Geometry: final body of the model. Coordinates: model frame, mm. Face numbers are marked on the shaded views. A direction names the side the tool comes from. Give positions to 0.01 mm unless a question says otherwise; leave off trailing zeros. Order: outer loops, then holes, each group sorted by start corner. A loop starts at its lowest first (then second) coordinate and runs counter-clockwise, first axis right, second up. Notation, with made-up numbers: (24.5, -25) - (63.5, -25) arc R27 ccw to (63.5, 10) - close; hole circle Ø5 at (50.5, 7). An arc over 180 degrees is marked (long way). Put each result on its own line as item: value. Start each with the question number.
1. Section C-C on y = -3.75. Return the cut outline in (x, z).
2. Set-up query: the marked faces 1 and 2. Return all of +Z, -Z, +X, -X, +Y, -Y with unobstructed straight access to the full face (end or side cutting, diameter ignored); none if empty.
3. First-contact query: P1, Ø1.5, axis at x = -2.5, y = -2, coming from the +Z side; P2, Ø3, axis at x = -2, y = -1, coming from the +Z side; P3, Ø2, axis at x = 2.5, z = -1.5, coming from the +Y side. Flat tips, straight axial feed; report the tip coordinate or a pass-through.
4. Section B-B on z = 0. Return the cut outline in (x, y), plus the area to 3 significant figures.
5. Section A-A on z = -5.5. Return the cut outline in (x, y), plus the area to 3 significant figures.
6. Ray query, line 1 along X through (y, z) = (-0.6, -2.25); line 2 along Y through (x, z) = (-2.75, 0). Return the intervals inside material, ascending. Write a range as from..to.
from build123d import *

# Parameters (mm, degrees)
F0_R      = 5.25
F1_DEPTH  = 4.6
F2_R      = 0.508
F4_DEPTH  = 0.2
F6_DEPTH  = 0.2
F7_W      = 0.2
F7_H      = 1
F8_DEPTH  = 1.7
F10_DEPTH = 0.2
F12_DEPTH = 0.2


with BuildPart() as f1:
    # F0 (on Front) → F1 (new body)
    with BuildSketch(Plane.XZ):
        Circle(F0_R)
    extrude(amount=F1_DEPTH)

    # F2
    f2_edges = [f1.edges().sort_by_distance(p)[0] for p in [
        (-5.25, -4.6, 0),
        (-5.25, 0, 0),
    ]]
    fillet(f2_edges, radius=F2_R)

    # F3 (on face) → F4 (join)
    with BuildSketch(Plane(origin=(0, 0, 0), x_dir=(-1, 0, 0), z_dir=(0, 1, 0))):
        with BuildLine():
            Line((0.8581771286, 0.338), (-0.8418228714, 0.338))
            Line((-0.8418228714, 0.338), (-0.8418228714, -4.6666795747))
            ThreePointArc((-0.8418228714, -4.6666795747), (-0.4225928635, -4.7231323581), (0, -4.742))
            ThreePointArc((0, -4.742), (0.430870892, -4.7223843844), (0.8581771286, -4.6636998205))
            Line((0.8581771286, -4.6636998205), (0.8581771286, 0.338))
        make_face()
        with BuildLine():
            ThreePointArc((0, -4.742), (-0.4225928635, -4.7231323581), (-0.8418228714, -4.6666795747))
            Line((-0.8418228714, -4.6666795747), (-0.8418228714, -4.742))
            Line((-0.8418228714, -4.742), (0, -4.742))
        make_face()
        with BuildLine():
            Line((0.8581771286, -4.742), (0.8581771286, -4.6636998205))
            ThreePointArc((0.8581771286, -4.6636998205), (0.430870892, -4.7223843844), (0, -4.742))
            Line((0, -4.742), (0.8581771286, -4.742))
        make_face()
    extrude(amount=F4_DEPTH)

    # F5 (on face) → F6 (join)
    with BuildSketch(Plane.XZ.offset(4.6)):
        with BuildLine():
            Line((-0.8581771286, -4.742), (0, -4.742))
            ThreePointArc((0, -4.742), (-0.430870892, -4.7223843844), (-0.8581771286, -4.6636998205))
            Line((-0.8581771286, -4.6636998205), (-0.8581771286, -4.742))
        make_face()
        with BuildLine():
            Line((0.8418228714, -4.6666795747), (0.8418228714, 0.338))
            Line((0.8418228714, 0.338), (-0.8581771286, 0.338))
            Line((-0.8581771286, 0.338), (-0.8581771286, -4.6636998205))
            ThreePointArc((-0.8581771286, -4.6636998205), (-0.430870892, -4.7223843844), (0, -4.742))
            ThreePointArc((0, -4.742), (0.4225928635, -4.7231323581), (0.8418228714, -4.6666795747))
        make_face()
        with BuildLine():
            Line((0.8418228714, -4.742), (0.8418228714, -4.6666795747))
            ThreePointArc((0.8418228714, -4.6666795747), (0.4225928635, -4.7231323581), (0, -4.742))
            Line((0, -4.742), (0.8418228714, -4.742))
        make_face()
    extrude(amount=F6_DEPTH)

    # F7 (on face) → F8 (join, through all)
    with BuildSketch(Plane.YZ.offset(0.8418228714)):
        with Locations((-4.8, -5.75)):
            Rectangle(F7_W, F7_H)
        with BuildLine():
            add(Edge.make_bspline(
                [(-4.8, -4.742), (-4.8333333333, -4.9113333333), (-4.901335109, -4.936598707), (-4.9, -5.25)],
                knots=[0, 0, 0, 0, 0.5177489739, 0.5177489739, 0.5177489739, 0.5177489739], degree=3))
            Line((-4.9, -5.25), (-4.7, -5.25))
            add(Edge.make_bspline(
                [(-4.6, -4.742), (-4.6333333333, -4.9113333333), (-4.7159921378, -4.9838428386), (-4.7, -5.25)],
                knots=[0, 0, 0, 0, 0.5177489739, 0.5177489739, 0.5177489739, 0.5177489739], degree=3))
            Line((-4.6, -4.742), (-4.8, -4.742))
        make_face()
        with Locations((0.2, -5.75)):
            Rectangle(F7_W, F7_H)
        with BuildLine():
            add(Edge.make_bspline(
                [(0, -4.742), (0.0333333333, -4.9113333333), (0.1159921378, -4.9838428386), (0.1, -5.25)],
                knots=[0, 0, 0, 0, 0.5177489739, 0.5177489739, 0.5177489739, 0.5177489739], degree=3))
            Line((0.1, -5.25), (0.3, -5.25))
            add(Edge.make_bspline(
                [(0.2, -4.742), (0.2333333333, -4.9113333333), (0.301335109, -4.936598707), (0.3, -5.25)],
                knots=[0, 0, 0, 0, 0.5177489739, 0.5177489739, 0.5177489739, 0.5177489739], degree=3))
            Line((0.2, -4.742), (0, -4.742))
        make_face()
    extrude(amount=-F8_DEPTH)

    # F9 (on face) → F10 (join, through all)
    with BuildSketch(Plane(origin=(0, 0.3, 0), x_dir=(-1, 0, 0), z_dir=(0, 1, 0))):
        with BuildLine():
            Line((0.4, -6.25), (-0.4, -6.25))
            Line((-0.4, -6.25), (-0.8418228714, -6.25))
            Line((-0.8418228714, -6.25), (-0.4735729361, -6.4726176162))
            ThreePointArc((-0.4735729361, -6.4726176162), (-0.4196612114, -6.5281834474), (-0.4, -6.6030665057))
            Line((-0.4, -6.6030665057), (-0.4, -9.0975669799))
            ThreePointArc((-0.4, -9.0975669799), (-0.3553534021, -9.2053534021), (-0.2475669799, -9.25))
            Line((-0.2475669799, -9.25), (0.2475669799, -9.25))
            ThreePointArc((0.2475669799, -9.25), (0.3553534021, -9.2053534021), (0.4, -9.0975669799))
            Line((0.4, -9.0975669799), (0.4, -6.6030665057))
            ThreePointArc((0.4, -6.6030665057), (0.4196612114, -6.5281834474), (0.4735729361, -6.4726176162))
            Line((0.4735729361, -6.4726176162), (0.8418228714, -6.25))
            Line((0.8418228714, -6.25), (0.4, -6.25))
        make_face()
    extrude(amount=-F10_DEPTH)

    # F11 (on face) → F12 (join, through all)
    with BuildSketch(Plane.XZ.offset(4.9)):
        with BuildLine():
            ThreePointArc((-0.4735729361, -6.4726176162), (-0.4196612114, -6.5281834474), (-0.4, -6.6030665057))
            Line((-0.4, -6.6030665057), (-0.4, -9.0975669799))
            ThreePointArc((-0.4, -9.0975669799), (-0.3553534021, -9.2053534021), (-0.2475669799, -9.25))
            Line((-0.2475669799, -9.25), (0.2475669799, -9.25))
            ThreePointArc((0.2475669799, -9.25), (0.3553534021, -9.2053534021), (0.4, -9.0975669799))
            Line((0.4, -9.0975669799), (0.4, -6.6030665057))
            ThreePointArc((0.4, -6.6030665057), (0.4196612114, -6.5281834474), (0.4735729361, -6.4726176162))
            Line((0.4735729361, -6.4726176162), (0.8418228714, -6.25))
            Line((0.8418228714, -6.25), (-0.8418228714, -6.25))
            Line((-0.8418228714, -6.25), (-0.4735729361, -6.4726176162))
        make_face()
    extrude(amount=-F12_DEPTH)


solid = f1.part
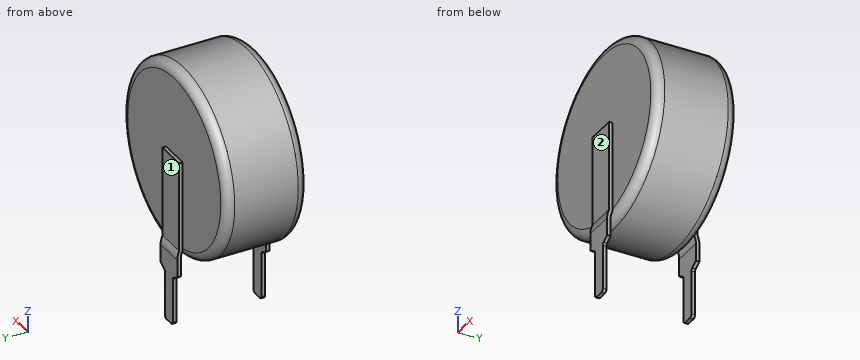
Resolved:
1. outline: circle Ø10.5 at (0, 0)
2. face 1: +Z, +X, -X, +Y
2. face 2: +Z, +X, -X, -Y
3. P1: z = 4.95
3. P2: z = 5.23
3. P3: y = 0
4. outline: (-5.25, -4.09) arc R0.51 ccw to (-4.74, -4.6) - (-0.86, -4.6) - (-0.86, -4.8) - (0.84, -4.8) - (0.84, -4.6) - (4.74, -4.6) arc R0.51 ccw to (5.25, -4.09) - (5.25, -0.51) arc R0.51 ccw to (4.74, 0) - (0.84, 0) - (0.84, 0.2) - (-0.86, 0.2) - (-0.86, 0) - (-4.74, 0) arc R0.51 ccw to (-5.25, -0.51) - close
4. area: 48.8 mm^2
5. outline: (-0.86, -4.9) - (0.84, -4.9) - (0.84, -4.7) - (-0.86, -4.7) - close; (-0.86, 0.1) - (0.84, 0.1) - (0.84, 0.3) - (-0.86, 0.3) - close
5. area: 0.680 mm^2
6. line 1: -4.74..4.74
6. line 2: -4.6..0
